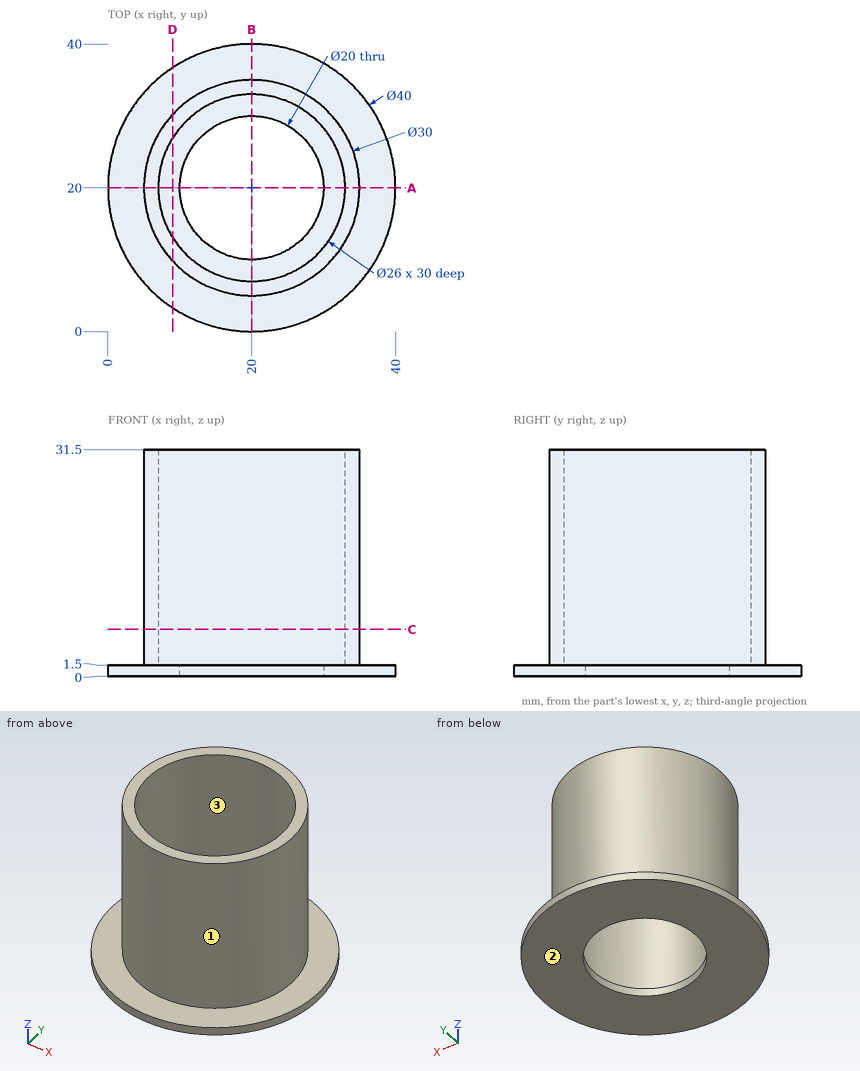
The drawing under review shows one solid part. Ordinate dimensions are in mm from its lowest x, y, z. Coordinates: 2 decimals unless noted, no trailing zeros. Loops run counter-clockwise (first coordinate to the right, second up) from the corner with the lowest first, then second, coordinate; pieces in that order, holes last. Notation, with made-up numbers: (0, 51) - (4, 51) arc R27 cw to (4, 84) - close; hole circle Ø10 at (79, -15). An arc over 180 degrees is marked (long way). Return JSON: item names as keys, results as strings.
Item 1: For line 1 (Y direction, x = 20, z = 0.5); line 2 (Y direction, x = 20, z = 15); line 3 (Z direction, x = 7.5, y = 11), list the stretches that pass through material, from the lowest coordinate up.
Determined:
{"line 1": "y = 0 to 10, 30 to 40", "line 2": "y = 5 to 7, 33 to 35", "line 3": "z = 0 to 1.5"}
Item 2: Take a section at A-A (y = 20). Give the boundary of the cut face in (x, z), then the cut area to 3 significant figures.
Determined:
{"outline": "(0, 0) - (10, 0) - (10, 1.5) - (7, 1.5) - (7, 31.5) - (5, 31.5) - (5, 1.5) - (0, 1.5) - close; (30, 0) - (40, 0) - (40, 1.5) - (35, 1.5) - (35, 31.5) - (33, 31.5) - (33, 1.5) - (30, 1.5) - close", "area": "150 mm2"}
Item 3: Insertion check: pin 1 (8 mm diameter, centred on x = 12, z = 6, fed in from -Y); pin 2 (4 mm diameter, centred on y = 17, z = 28, fed in from -X); pin 3 (2 mm diameter, centred on y = 24, z = 9, fed in from -X); pin 4 (4 mm diameter, centred on x = 4.5, y = 4, fed in from +Z). Each pin has a flat end and moves straight along its axis. Give the tip position at first contact, or say it passes through.
Determined:
{"pin 1": "stops at y = 5.54", "pin 2": "stops at x = 5.03", "pin 3": "stops at x = 5.3", "pin 4": "passes through"}
Item 4: Mouldability with a two-part tool opening along X and no side actions: class the marked faces 1, 2 and 3 as pulls with the +X half, pulls with the -X half, needs draft (parallel to the pull), parting line crosses it, or undercut.
Determined:
{"face 1": "parting line crosses it", "face 2": "needs draft", "face 3": "undercut"}
Item 5: Take a section at C-C (z = 6.5). Give the boundary of the cut face in (x, y).
Determined:
{"outline": "circle Ø30 at (20, 20); hole circle Ø26 at (20, 20)"}
Item 6: Take a section at D-D (x = 9). Give the boundary of the cut face in (y, z), then the cut area to 3 significant figures.
Determined:
{"outline": "(3.3, 0) - (36.7, 0) - (36.7, 1.5) - (30.2, 1.5) - (30.2, 31.5) - (26.93, 31.5) - (26.93, 1.5) - (13.07, 1.5) - (13.07, 31.5) - (9.8, 31.5) - (9.8, 1.5) - (3.3, 1.5) - close", "area": "246 mm2"}
